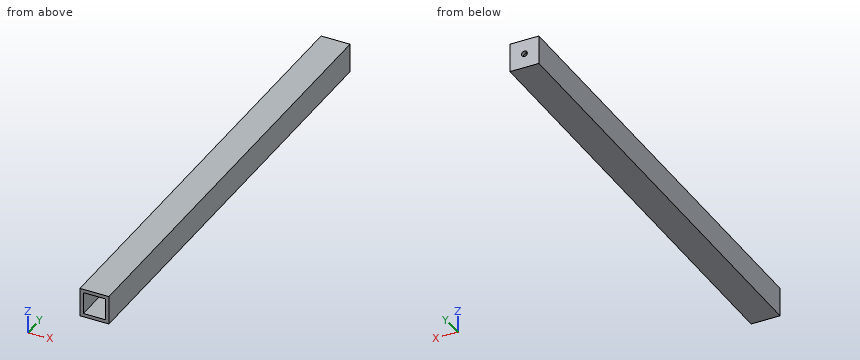
from build123d import *

# Parameters (mm, degrees)
SKETCH1_W           = 25
SKETCH1_H           = 25
BOSS_EXTRUDE1_DEPTH = 400
SHELL1_T            = -3
SKETCH2_W           = 19
SKETCH2_H           = 19
SKETCH2_R           = 2.5
BOSS_EXTRUDE2_DEPTH = 3


with BuildPart() as part:
    # Sketch1 → Boss-Extrude1 (new body)
    with BuildSketch(Plane(origin=(0, 0, 0), x_dir=(1, 0, 0), z_dir=(0, 1, 0))):
        Rectangle(SKETCH1_W, SKETCH1_H)
    extrude(amount=BOSS_EXTRUDE1_DEPTH)

    # Shell1
    shell1_openings = [part.faces().sort_by_distance(p)[0] for p in [
        (0, 400, 0),
        (0, 0, 0),
    ]]
    offset(amount=SHELL1_T, openings=shell1_openings, kind=Kind.INTERSECTION)

    # Sketch2 → Boss-Extrude2 (add)
    with BuildSketch(Plane(origin=(0, 400, 0), x_dir=(1, 0, 0), z_dir=(0, 1, 0))):
        Rectangle(SKETCH2_W, SKETCH2_H)
        Circle(SKETCH2_R, mode=Mode.SUBTRACT)
    extrude(amount=-BOSS_EXTRUDE2_DEPTH)


solid = part.part
CAD build for the part. Positions are in the model's coordinates, mm. Coordinates: 2 decimals unless noted, no trailing zeros. Order: outer loops, then holes, each group sorted by start corner. A loop starts at its lowest first (then second) coordinate and runs counter-clockwise, first axis right, second up. Notation, with made-up numbers: (2.5, 30.5) -> (43.5, 30.5) arc R24 cw to (43.5, 58.5) -> close; hole circle Ø7 at (15, 31). An arc over 180 degrees is marked (long way). Answer in a Markdown table with one row per item.
1) Drill centre lines: line 1 (X direction, y = 270, z = 3); line 2 (X direction, y = 398.35, z = 0). Where is each one in solid material? Low to high.
Check values:
| item | result |
|---|---|
| line 1 | -12.5 to -9.5, 9.5 to 12.5 |
| line 2 | -12.5 to -2.5, 2.5 to 12.5 |
2) Band-saw the part on B-B (z = 6.25). List the corners of the cut face in (x, y).
Check values:
| item | result |
|---|---|
| outline | (-12.5, 0) -> (-9.5, 0) -> (-9.5, 397) -> (9.5, 397) -> (9.5, 0) -> (12.5, 0) -> (12.5, 400) -> (-12.5, 400) -> close |
3) Band-saw the part on A-A (y = 81). List the corners of the cut face in (x, z), and give its area (3 significant figures).
Check values:
| item | result |
|---|---|
| outline | (-12.5, -12.5) -> (12.5, -12.5) -> (12.5, 12.5) -> (-12.5, 12.5) -> close; hole (-9.5, -9.5) -> (9.5, -9.5) -> (9.5, 9.5) -> (-9.5, 9.5) -> close |
| area | 264 mm2 |
4) Flat gauge pins, fed straight in: P1, Ø4.5, axis at x = 0, z = 0, coming from the +Y side; P2, Ø9.5, axis at x = 4, z = 4, coming from the -Y side. Where does each tip first touch, or does it go through?
Check values:
| item | result |
|---|---|
| P1 | through |
| P2 | y = 397 |
